```python
from build123d import *

# Parameters (mm, degrees)
F1_DEPTH = 10
F2_R     = 7


with BuildPart() as f1:
    # F0 (on Top) → F1 (new body)
    with BuildSketch(Plane.XY):
        with BuildLine():
            Line((-5.2952272627, 38.5407575913), (-13.4240464083, 25.8959278094))
            ThreePointArc((-13.4240464083, 25.8959278094), (-13.8750817001, 24.9329216495), (-14.0564356508, 23.8851027514))
            add(Edge.make_bspline(
                [(-14.0564356508, 23.8851027514), (-13.8623993356, 19.7947937773), (-13.2387703053, 11.566177165), (-7.8025218047, 2.478450576), (-1.7911023938, 0.6541447849), (0, 0)],
                knots=[0, 0, 0, 0, 0.3727156088, 0.7096918573, 1, 1, 1, 1], degree=3))
            add(Edge.make_bspline(
                [(14.0564356508, 23.8851027514), (13.8623993356, 19.7947937773), (13.2387703053, 11.566177165), (7.8025218047, 2.478450576), (1.7911023938, 0.6541447849), (0, 0)],
                knots=[0, 0, 0, 0, 0.3727156088, 0.7096918573, 1, 1, 1, 1], degree=3))
            ThreePointArc((14.0564356508, 23.8851027514), (13.8750817001, 24.9329216495), (13.4240464083, 25.8959278094))
            Line((13.4240464083, 25.8959278094), (5.2952272627, 38.5407575913))
            ThreePointArc((5.2952272627, 38.5407575913), (4.9332368552, 38.8777122511), (4.4540487874, 39))
            Line((4.4540487874, 39), (-4.4540487874, 39))
            ThreePointArc((-4.4540487874, 39), (-4.9332368552, 38.8777122511), (-5.2952272627, 38.5407575913))
        make_face()
    extrude(amount=F1_DEPTH)

    # F2
    f2_edges = [f1.edges().sort_by_distance(p)[0] for p in [
        (0, 0, 5),
    ]]
    fillet(f2_edges, radius=F2_R)


solid = f1.part
```
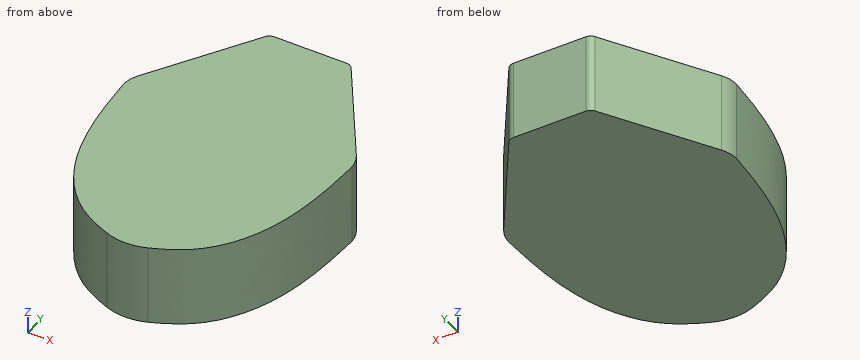
Work out the finished part from the listing and answer in its coordinate system (mm). Coordinates: 2 decimals unless noted, no trailing zeros. Loops run counter-clockwise (first coordinate to the right, second up) from the corner with the lowest first, then second, coordinate; pieces in that order, holes last.
1) Flat-ended cylindrical pins translate along their axes: pin 1 (3 mm diameter, centred on y = 6, z = 1, fed in from +X); pin 2 (5 mm diameter, centred on x = 6.5, y = 5, fed in from -Z); pin 3 (1 mm diameter, centred on x = -8, z = 3.5, fed in from +Y); pin 4 (1 mm diameter, centred on y = 10.5, z = 5, fed in from +X). Find the tip coordinate at first contact, or state that the pin passes through.
Results:
pin 1: stops at x = 10.51
pin 2: stops at z = 0
pin 3: stops at y = 35.11
pin 4: stops at x = 12.1
2) Consider probe 1 along Y at (x, z) = (-0.25, 5.5); probe 2 along X at (y, z) = (22, 1.5); probe 3 along X at (y, z) = (31.5, 3.75). Determine where each line is inside the solid, lowest interval first.
Results:
probe 1: y = 0.45 to 39
probe 2: x = -13.96 to 13.96
probe 3: x = -9.82 to 9.82
3) Section A-A (y = 31) is taken. Give the vertices of the cut face in (x, z), plus the area to 3 significant figures.
Results:
outline: (-10.14, 0) - (10.14, 0) - (10.14, 10) - (-10.14, 10) - close
area: 203 mm2
